from build123d import *

# Parameters (mm, degrees)
BOSS_EXTRUDE1_DEPTH = 37
CUT_EXTRUDE1_DEPTH  = 32.5


with BuildPart() as part:
    # Sketch1 → Boss-Extrude1 (new body)
    with BuildSketch(Plane.XY):
        with BuildLine():
            Line((40.356535193, -22.947426174), (22.947426174, -40.356535193))
            ThreePointArc((22.947426174, -40.356535193), (15.156681171, -45.914203278), (5.981257322, -48.63357442))
            ThreePointArc((5.981257322, -48.63357442), (0, -49), (-5.981257322, -48.63357442))
            ThreePointArc((-5.981257322, -48.63357442), (-15.156681171, -45.914203278), (-22.947426174, -40.356535193))
            Line((-22.947426174, -40.356535193), (-40.356535193, -22.947426174))
            ThreePointArc((-40.356535193, -22.947426174), (-45.914203278, -15.156681171), (-48.63357442, -5.981257322))
            ThreePointArc((-48.63357442, -5.981257322), (-42.907888217, 23.662483572), (-20.892307913, 44.322809817))
            ThreePointArc((-20.892307913, 44.322809817), (-19.322951214, 44.702303901), (-17.73141344, 44.430451502))
            ThreePointArc((-17.73141344, 44.430451502), (-12.910393927, 43.910800792), (-8.488178405, 45.899839725))
            ThreePointArc((-8.488178405, 45.899839725), (0.386708758, 48.850803922), (9.16390657, 45.62084875))
            ThreePointArc((9.16390657, 45.62084875), (13.572775182, 43.625772556), (18.385878971, 44.128249799))
            ThreePointArc((18.385878971, 44.128249799), (20.002215513, 44.392928913), (21.589134046, 43.987603835))
            ThreePointArc((21.589134046, 43.987603835), (43.093258956, 23.323186587), (48.63357442, -5.981257322))
            ThreePointArc((48.63357442, -5.981257322), (45.914203278, -15.156681171), (40.356535193, -22.947426174))
        make_face()
    extrude(amount=BOSS_EXTRUDE1_DEPTH)

    # Sketch3 → Cut-Extrude1 (cut)
    with BuildSketch(Plane.XY.offset(37)):
        with BuildLine():
            Line((-39.649428412, -22.240319392), (-22.240319392, -39.649428412))
            ThreePointArc((-22.240319392, -39.649428412), (-14.718220769, -45.015452769), (-5.859190846, -47.641052493))
            ThreePointArc((-5.859190846, -47.641052493), (0, -48), (5.859190846, -47.641052493))
            ThreePointArc((5.859190846, -47.641052493), (14.718220769, -45.015452769), (22.240319392, -39.649428412))
            Line((22.240319392, -39.649428412), (39.649428412, -22.240319392))
            ThreePointArc((39.649428412, -22.240319392), (45.015452769, -14.718220769), (47.641052493, -5.859190846))
            ThreePointArc((47.641052493, -5.859190846), (42.213804691, 22.847203188), (21.148539474, 43.089897634))
            ThreePointArc((21.148539474, 43.089897634), (19.958350574, 43.393891443), (18.746098167, 43.195382107))
            ThreePointArc((18.746098167, 43.195382107), (13.413001918, 42.638618817), (8.52781313, 44.849236713))
            ThreePointArc((8.52781313, 44.849236713), (0.378047137, 47.850813988), (-7.865478644, 45.117238565))
            ThreePointArc((-7.865478644, 45.117238565), (-12.761098878, 42.921980343), (-18.095263428, 43.498993941))
            ThreePointArc((-18.095263428, 43.498993941), (-19.288916758, 43.702883241), (-20.465934283, 43.418262678))
            ThreePointArc((-20.465934283, 43.418262678), (-42.032217029, 23.179575744), (-47.641052493, -5.859190846))
            ThreePointArc((-47.641052493, -5.859190846), (-45.015452769, -14.718220769), (-39.649428412, -22.240319392))
        make_face()
    extrude(amount=-CUT_EXTRUDE1_DEPTH, mode=Mode.SUBTRACT)


solid = part.part
Model file for the job. Use its own axes, mm. A direction names the side the tool comes from. Coordinates: 2 decimals unless noted, no trailing zeros. Order: outer loops, then holes, each group sorted by start corner. A loop starts at its lowest first (then second) coordinate and runs counter-clockwise, first axis right, second up. Notation, with made-up numbers: (44.25, 78.25) -> (54.25, 78.25) arc R32 ccw to (54.25, 112.25) -> close; hole circle Ø1 at (88, -38). An arc over 180 degrees is marked (long way). Return JSON: item names as keys, results as strings. Group by question number.
Item 1: Saw through at A-A on x = -29.5. Write the cut outline in (y, z), then the cut area to 3 significant figures.
Item 2: Tool access for faces 1 (the flat face through (31.774, -31.53, 18.241)), 2 (the flat face through (30.82, -31.07, 20.98)): list every direction of +Z, -Z, +X, -X, +Y, -Y with a clear straight run to the whole face (end or side of a thin tool).
Item 3: Wall check: line 1 along Z through (x, y) = (18, -28); line 2 along X through (y, z) = (28.5, 23); line 3 along X through (y, z) = (19, 10). Give the ranges that are in metal, low to high. Write a range as [from, to].
Item 4: Saw through at C-C on y = -17. Write the cut outline in (x, z).
Item 5: Saw through at B-B on z = 6. Write the cut outline in (x, y), then the cut area to 3 significant figures.
Item 6: Flat gauge pins, fed straight in: P1, Ø8, axis at x = -38, y = -5.5, coming from the +Z side; P2, Ø1.5, axis at y = -23.5, z = 4, coming from the +X side; P3, Ø1.5, axis at y = 30.5, z = 22, coming from the +X side. Where does each tip first touch, or does it go through?
Item 7: Pull direction X, two halves, no side cores. Call faces 3 (the cylindrical face through (45.97, -15.04, 18.24)), 4 (the flat face through (-1, 1, 4.5)), 5 (the cylindrical face through (0, -49, 18)): pulls with the +X half, pulls with the -X half, needs draft (parallel to the pull), parting line crosses it, or undercut.
Values found:
{
 "1": {"outline": "(-33.8, 0) -> (39.12, 0) -> (39.12, 37) -> (37.86, 37) -> (37.86, 4.5) -> (-32.39, 4.5) -> (-32.39, 37) -> (-33.8, 37) -> close", "area": "415 mm2"},
 "2": {"face 1": "+Z, -Z, +X, -Y", "face 2": "+Z"},
 "3": {"line 1": "z = [0, 4.5]", "line 2": "x = [-39.86, -38.62], [38.62, 39.86]", "line 3": "x = [-45.17, -44.08], [44.08, 45.17]"},
 "4": {"outline": "(-44.93, 0) -> (44.93, 0) -> (44.93, 37) -> (43.77, 37) -> (43.77, 4.5) -> (-43.77, 4.5) -> (-43.77, 37) -> (-44.93, 37) -> close"},
 "5": {"outline": "(-48.63, -5.98) arc R29 ccw to (-40.36, -22.95) -> (-22.95, -40.36) arc R29 ccw to (-5.98, -48.63) arc R49 ccw to (5.98, -48.63) arc R29 ccw to (22.95, -40.36) -> (40.36, -22.95) arc R29 ccw to (48.63, -5.98) arc R49 ccw to (21.59, 43.99) arc R4 ccw to (18.39, 44.13) arc R9.26 cw to (9.16, 45.62) arc R14.15 ccw to (-8.49, 45.9) arc R9.26 cw to (-17.73, 44.43) arc R4 ccw to (-20.89, 44.32) arc R49 ccw to start; hole (-47.64, -5.86) arc R28 ccw to (-39.65, -22.24) -> (-22.24, -39.65) arc R28 ccw to (-5.86, -47.64) arc R48 ccw to (5.86, -47.64) arc R28 ccw to (22.24, -39.65) -> (39.65, -22.24) arc R28 ccw to (47.64, -5.86) arc R48 ccw to (21.15, 43.09) arc R3 ccw to (18.75, 43.2) arc R10.26 cw to (8.53, 44.85) arc R13.15 ccw to (-7.87, 45.12) arc R10.26 cw to (-18.1, 43.5) arc R3 ccw to (-20.47, 43.42) arc R48 ccw to start", "area": "302 mm2"},
 "6": {"P1": "stops at z = 4.5", "P2": "stops at x = 40.55", "P3": "stops at x = 38.94"},
 "7": {"face 3": "pulls with the +X half", "face 4": "undercut", "face 5": "parting line crosses it"}
}
